The model under review builds one solid part; all positions refer to its coordinate system, in mm. Face numbers are marked on the shaded views. A direction names the side the tool comes from. Coordinates: 2 decimals unless noted, no trailing zeros. Write each loop counter-clockwise with the first axis right and the second up, starting at its lowest first coordinate (ties: lowest second). Pieces come first, ordered by that corner, then holes. Notation, with made-up numbers: M -4,28.25 L 24,28.25 A24 ccw 24,67.25 Z; hole C 64.5,-12 d1. An arc over 180 degrees is marked long. Answer as a JSON object with one key per item and string values.
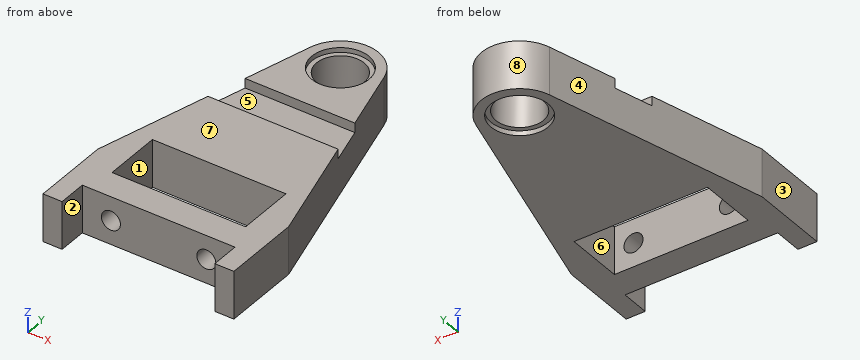
```python
from build123d import *

# Parameters (mm, degrees)
SKETCH1_R           = 25
SKETCH1_W           = 140
SKETCH1_H           = 60
BOSS_EXTRUDE1_DEPTH = 25
SKETCH4_R           = 30
CUT_EXTRUDE1_DEPTH  = 5
CUT_EXTRUDE2_DEPTH  = 10
CUT_EXTRUDE3_REACH  = 312
SKETCH6_R           = 10


with BuildPart() as part:
    # Sketch1 → Boss-Extrude1 (new body, symmetric)
    with BuildSketch(Plane.XY):
        with BuildLine():
            Line((100, 81.343051449), (38.637033052, 310.352761804))
            ThreePointArc((38.637033052, 310.352761804), (0, 340), (-38.637033052, 310.352761804))
            Line((-38.637033052, 310.352761804), (-100, 81.343051449))
            Line((-100, 81.343051449), (-100, 0))
            Line((-100, 0), (-80, 0))
            Line((-80, 0), (-80, 30))
            Line((-80, 30), (80, 30))
            Line((80, 30), (80, 0))
            Line((80, 0), (100, 0))
            Line((100, 0), (100, 81.343051449))
        make_face()
        with Locations((0, 300)):
            Circle(SKETCH1_R, mode=Mode.SUBTRACT)
        with Locations((0, 90)):
            Rectangle(SKETCH1_W, SKETCH1_H, mode=Mode.SUBTRACT)
    extrude(amount=BOSS_EXTRUDE1_DEPTH, both=True)

    # Sketch4 → Cut-Extrude1 (cut)
    with BuildSketch(Plane.XY.offset(25)):
        with Locations((0, 300)):
            Circle(SKETCH4_R)
    cut_extrude1 = extrude(amount=-CUT_EXTRUDE1_DEPTH, mode=Mode.SUBTRACT)

    # Mirror1: Cut-Extrude1 across plane
    add(cut_extrude1.mirror(Plane.XY), mode=Mode.SUBTRACT)

    # Sketch5 → Cut-Extrude2 (cut)
    with BuildSketch(Plane.XY.offset(25)):
        Polygon((-57.487998762, 240), (57.487998762, 240), (68.20596646, 200), (-68.20596646, 200), align=None)
    extrude(amount=-CUT_EXTRUDE2_DEPTH, mode=Mode.SUBTRACT)

    # Sketch6 → Cut-Extrude3 (cut, up to next)
    with BuildSketch(Plane.XZ.offset(-30), mode=Mode.PRIVATE) as cut_extrude3_sk1:
        with Locations((-50, 0)):
            Circle(SKETCH6_R)
    cut_extrude3_tool1 = extrude(cut_extrude3_sk1.sketch, amount=-CUT_EXTRUDE3_REACH, mode=Mode.PRIVATE) & part.part
    add(cut_extrude3_tool1.solids().sort_by_distance((-50, 30, 0))[0], mode=Mode.SUBTRACT)
    # Sketch6 → Cut-Extrude3 (cut, up to next)
    with BuildSketch(Plane.XZ.offset(-30), mode=Mode.PRIVATE) as cut_extrude3_sk2:
        with Locations((50, 0)):
            Circle(SKETCH6_R)
    cut_extrude3_tool2 = extrude(cut_extrude3_sk2.sketch, amount=-CUT_EXTRUDE3_REACH, mode=Mode.PRIVATE) & part.part
    add(cut_extrude3_tool2.solids().sort_by_distance((50, 30, 0))[0], mode=Mode.SUBTRACT)


solid = part.part
```
(1) Add section A-A on z = 0. Give the boundary of the cut face in (x, y), and give its area (3 significant figures).
Results list:
{"outline": "M -100,0 L -80,0 L -80,30 L -60,30 L -60,60 L -70,60 L -70,120 L 70,120 L 70,60 L 60,60 L 60,30 L 80,30 L 80,0 L 100,0 L 100,81.34 L 38.64,310.35 A40 ccw -38.64,310.35 L -100,81.34 Z; M -40,30 L 40,30 L 40,60 L -40,60 Z; hole C 0,300 d50", "area": "33,300 mm²"}
(2) Add section C-C on x = 0. Give the boundary of the cut face in (y, z), and give its area (3 significant figures).
Results list:
{"outline": "M 30,-25 L 60,-25 L 60,25 L 30,25 Z; M 120,-25 L 270,-25 L 270,-20 L 275,-20 L 275,20 L 270,20 L 270,25 L 240,25 L 240,15 L 200,15 L 200,25 L 120,25 Z; M 325,-20 L 330,-20 L 330,-25 L 340,-25 L 340,25 L 330,25 L 330,20 L 325,20 Z", "area": "9,500 mm²"}
(3) Add section B-B on z = -14. Give the boundary of the cut face in (x, y).
Results list:
{"outline": "M -100,0 L -80,0 L -80,30 L 80,30 L 80,0 L 100,0 L 100,81.34 L 38.64,310.35 A40 ccw -38.64,310.35 L -100,81.34 Z; hole M -70,60 L 70,60 L 70,120 L -70,120 Z; hole C 0,300 d50"}
(4) Wall thickness on line 1 along X through (y, z) = (52, -2); line 2 along Y through (x, z) = (22, -18); line 3 along Z through (x, y) = (-50, 39): over which ranges is each line inside the solid? List them lowest first. Write a range as from..to.
Results list:
{"line 1": "-100..-59.8, -40.2..40.2, 59.8..100", "line 2": "30..60, 120..288.13, 311.87..333.41", "line 3": "-25..-10, 10..25"}
(5) Draft analysis for pull direction X (two halves, no side actions). For the marked faces 6, 7 and 8, state which applies: released by +X, released by -X, zero draft, split by the parting line, or undercut.
Results list:
{"face 6": "undercut", "face 7": "zero draft", "face 8": "split by the parting line"}
(6) Add section D-D on x = -34. Give the boundary of the cut face in (y, z), and give its area (3 significant figures).
Results list:
{"outline": "M 30,-25 L 60,-25 L 60,25 L 30,25 Z; M 120,-25 L 321.07,-25 L 321.07,25 L 240,25 L 240,15 L 200,15 L 200,25 L 120,25 Z", "area": "11,200 mm²"}
(7) For pin 1 Ø5 at (x, z) = (6.5, 18) entering from -Y; pin 2 Ø25 at (y, z) = (89.5, 6.5) entering from -X; pin 3 Ø12 at (x, z) = (50, 0) entering from -Y; pin 4 Ø1 at (y, z) = (179, -18.5) entering from -X, all flat-tipped, find the tip position at first contact; note any pin that passes through.
Results list:
{"pin 1": "y = 30", "pin 2": "x = -100", "pin 3": "y = 120", "pin 4": "x = -73.97"}
(8) For the marked faces 1, 2, 3, 4 and 5, list the 3-axis set-ups (+Z, -Z, +X, -X, +Y, -Y) from which the entire face can be reached by the end or side of a thin tool; tool diameter is ignored.
Results list:
{"face 1": "+Z, -Z", "face 2": "+Z, -Z, -Y", "face 3": "+Z, -Z, -X, +Y, -Y", "face 4": "+Z, -Z, -X, +Y", "face 5": "+Z, +X, -X"}
